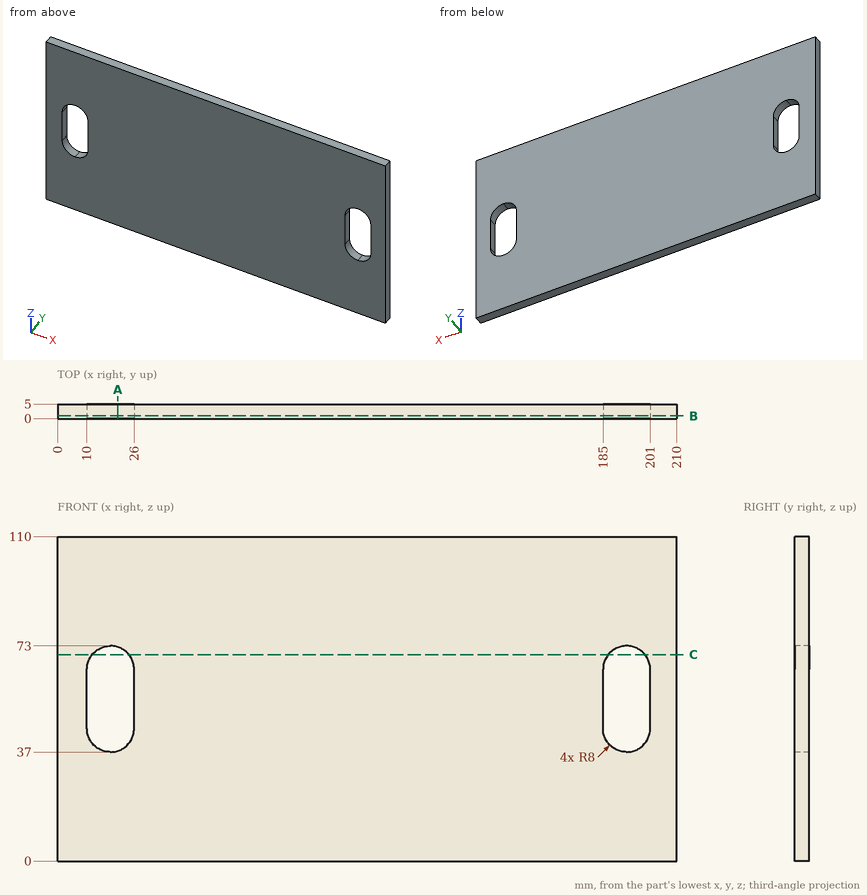
For this review, use the dimensioned drawing (mm, ordinates from the lowest corner) and the shaded views. Round coordinates to 2 decimals unless told otherwise and drop trailing zeros. Write each loop counter-clockwise with the first axis right and the second up, starting at its lowest first coordinate (ties: lowest second). Pieces come first, ordered by that corner, then holes. Notation, with made-up numbers: (71, 53.25) - (122, 53.25) arc R20 cw to (122, 81.25) - close; hole circle Ø5 at (58, -26.75). An arc over 180 degrees is marked (long way). Use a Markdown table: item, result.
Q1. We need section A-A (x = 20.5). Give the boundary of the cut face in (y, z), plus the area to 3 significant figures.
Derived:
| item | result |
|---|---|
| outline | (0, 0) - (5, 0) - (5, 37.4) - (0, 37.4) - close; (0, 72.6) - (5, 72.6) - (5, 110) - (0, 110) - close |
| area | 374 mm2 |
Q2. We need section B-B (y = 0.95). State how many separate pieces and enclosed holes the cut face has, plus the area to 3 significant figures.
Derived:
| item | result |
|---|---|
| separate pieces | 1 |
| enclosed holes | 2 |
| area | 22,100 mm2 |
Q3. Wall thickness on line 1 along X through (y, z) = (2.6, 57.5); line 2 along X through (y, z) = (1.8, 67); line 3 along Z through (x, y) = (21.5, 1.2): over which ranges is each line inside the solid? List them lowest first.
Derived:
| item | result |
|---|---|
| line 1 | x = 0 to 10, 26 to 185, 201 to 210 |
| line 2 | x = 0 to 10.25, 25.75 to 185.25, 200.75 to 210 |
| line 3 | z = 0 to 37.81, 72.19 to 110 |
Q4. We need section C-C (z = 70). Give the boundary of the cut face in (x, y) (3 decimals).
Derived:
| item | result |
|---|---|
| outline | (0, 0) - (11.755, 0) - (11.755, 5) - (0, 5) - close; (24.245, 0) - (186.755, 0) - (186.755, 5) - (24.245, 5) - close; (199.245, 0) - (210, 0) - (210, 5) - (199.245, 5) - close |
